Source: CAD feature listing. Evaluate the final solid. Frame: model axes, mm. A direction names the side the tool comes from. Coordinates: 2 decimals unless noted, no trailing zeros. Write each loop counter-clockwise with the first axis right and the second up, starting at its lowest first coordinate (ties: lowest second). Pieces come first, ordered by that corner, then holes. Notation, with made-up numbers: (76.5, -25) - (112.5, -25) arc R14 ccw to (112.5, 1) - close; hole circle Ø10 at (-6.5, 16). An arc over 180 degrees is marked (long way). One line per item, written item: value.
from build123d import *

# Parameters (mm, degrees)
BOSS_EXTRUDE3_DEPTH = 13
FILLET1_R           = 1
FILLET2_R           = 5
SKETCH2_R           = 2.4
CUT_EXTRUDE1_DEPTH  = 7.5
FILLET3_R           = 2.5


with BuildPart() as part:
    # Sketch1 → Boss-Extrude3 (new body)
    with BuildSketch(Plane.XY):
        Polygon((-12.5, 10.5), (-4.45, 10.5), (4.45, 10.5), (12.5, 10.5), (12.5, 24.5), (-12.5, 33.7), align=None)
        Polygon((-4.45, 7.3), (-10.25, 7.3), (-4, 0), (4, 0), (10.25, 7.3), (4.45, 7.3), (4.45, 10.5), (-4.45, 10.5), align=None)
        Polygon((-15.5, 34.804), (-12.5, 33.7), (-12.5, 10.5), (-15.5, 10.5), align=None)
    extrude(amount=BOSS_EXTRUDE3_DEPTH)

    # Fillet1
    fillet1_edges = [part.edges().sort_by_distance(p)[0] for p in [
        (10.25, 7.3, 6.5),
        (-10.25, 7.3, 6.5),
    ]]
    fillet(fillet1_edges, radius=FILLET1_R)

    # Fillet2
    fillet2_edges = [part.edges().sort_by_distance(p)[0] for p in [
        (4, 0, 6.5),
        (-4, 0, 6.5),
    ]]
    fillet(fillet2_edges, radius=FILLET2_R)

    # Sketch2 → Cut-Extrude1 (cut)
    with BuildSketch(Plane(origin=(9.431542754, 25.629192267, 0), x_dir=(0.9384712337524266, -0.3453574140208928, 0), z_dir=(0.3453574140208928, 0.9384712337524266, 0))):
        with Locations(Location((-20.450055857, -6.5, 0), (0, 0, 180))):
            Circle(SKETCH2_R)
        with Locations(Location((-5.450055857, -6.5, 0), (0, 0, 180))):
            Circle(SKETCH2_R)
    extrude(amount=-CUT_EXTRUDE1_DEPTH, mode=Mode.SUBTRACT)

    # Fillet3
    fillet3_edges = [part.edges().sort_by_distance(p)[0] for p in [
        (-15.5, 22.652, 13),
        (-15.5, 22.652, 0),
        (12.5, 17.5, 0),
        (12.5, 17.5, 13),
    ]]
    fillet(fillet3_edges, radius=FILLET3_R)


solid = part.part
1) Material intervals for line 1 (X direction, y = 10, z = 12.25); line 2 (Y direction, x = 8.5, z = 1); line 3 (Z direction, x = 3.25, y = 20.5), sorted ascending.
Values found:
line 1: -4.45 to 4.45
line 2: 5.26 to 7.21, 10.5 to 25.97
line 3: 0 to 4.57, 8.43 to 13
2) Draft query along X for faces 1 (the flat face through (-1.3, 29.58, 6.41)), 2 (the flat face through (-4.45, 9, 6)), 3 (the cylindrical face through (5.29, 23.21, 6.61)), 4 (the flat face through (-10, 10.5, 6)). Return one class per face: released by +X, released by -X, zero draft, split by the parting line, or undercut.
Values found:
face 1: released by +X
face 2: released by -X
face 3: undercut
face 4: zero draft
3) Section query B-B on x = -6. Output: boundary loops of the cut face in (y, z).
Values found:
outline: (2.34, 0) - (7.3, 0) - (7.3, 13) - (2.34, 13) - close; (10.5, 0) - (31.31, 0) - (31.31, 13) - (10.5, 13) - close
4) Contact query for flat-ended pins moving along their axis: P1, Ø3, axis at x = 6, z = 4, coming from the +Y side; P2, Ø1.1, axis at x = -7, z = 3.5, coming from the +Y side; P3, Ø1.6, axis at y = 9, z = 3.5, coming from the -X side. Output: stop coordinate, or through.
Values found:
P1: y = 27.44
P2: y = 31.88
P3: x = -4.45
5) Reachability of faces 5 (the flat face through (-6, 7.3, 6)), 6 (the flat face through (4.45, 9, 6)), 7 (the flat face through (-12.32, 25.64, 6.53)) from +Z, -Z, +X, -X, +Y, -Y: full face, straight path, thin tool, end or side. Return the list, or none.
Values found:
face 5: +Z, -Z, -X
face 6: +Z, -Z, +X
face 7: none
6) Section query D-D on x = 10.5. Output: boundary loops of the cut face in (y, z).
Values found:
outline: (10.5, 0.05) - (25.24, 0.05) - (25.24, 12.95) - (10.5, 12.95) - close
7) Section query C-C on y = 9. Output: boundary loops of the cut face in (x, z).
Values found:
outline: (-4.45, 0) - (4.45, 0) - (4.45, 13) - (-4.45, 13) - close
8) Section query A-A on z = 3.25. Output: boundary loops of the cut face in (x, y), then the cut area to 3 significant figures.
Values found:
outline: (-15.5, 10.5) - (-4.45, 10.5) - (-4.45, 7.3) - (-8.08, 7.3) arc R1 ccw to (-8.84, 5.65) - (-5.5, 1.75) arc R5 ccw to (-1.7, 0) - (1.7, 0) arc R5 ccw to (5.5, 1.75) - (8.84, 5.65) arc R1 ccw to (8.08, 7.3) - (4.45, 7.3) - (4.45, 10.5) - (12.5, 10.5) - (12.5, 24.5) - (-15.5, 34.8) - close
area: 665 mm2
